Geometry: final body of the model. Coordinates: model frame, mm. Face numbers are marked on the shaded views. A direction names the side the tool comes from. Give positions to 0.01 mm unless a question says otherwise; leave off trailing zeros. Write each loop counter-clockwise with the first axis right and the second up, starting at its lowest first coordinate (ties: lowest second). Pieces come first, ordered by that corner, then holes. Notation, with made-up numbers: (60, -1.5) - (84, -1.5) arc R11 cw to (84, 14.5) - close; hole circle Ø7 at (20, 14). An arc over 180 degrees is marked (long way). Use CSV: the item, a comma, the result in double quotes. Start each with the question number.
(1) Section D-D on y = 23. Output: boundary loops of the cut face in (x, z), and give its area (3 significant figures).
(2) First-contact query: pin 1 Ø1.5 at (x, y) = (-15.5, 48.5) entering from +Z; pin 2 Ø10 at (y, z) = (23.5, 8) entering from -X; pin 3 Ø2 at (x, z) = (-3, -15.5) entering from +Y; pin 4 Ø4 at (y, z) = (7.5, -24.5) entering from -X. Flat tips, straight axial feed; report the tip coordinate or a pass-through.
(3) Draft query along Y for the marked faces 1, 2 and 3. Return one class per face: released by +Y, released by -Y, zero draft, split by the parting line, or undercut.
(4) Section A-A on z = -24. Output: boundary loops of the cut face in (x, y).
(5) Section C-C on x = 0. Output: boundary loops of the cut face in (y, z), and give its area (3 significant figures).
(6) Line query: probe 1 along Y at (x, z) = (-17.5, 5.5); probe 2 along Z at (x, y) = (4, 13.5); probe 3 along Y at (x, z) = (10, 0). Output: solid intervals per line, ascending. Write a range as [from, to].
(7) Reachability of the marked faces 4, 5, 6 and 7 from +Z, -Z, +X, -X, +Y, -Y: full face, straight path, thin tool, end or side. Return the list, or none.
(8) Section B-B on z = 0. Output: boundary loops of the cut face in (x, y), and give its area (3 significant figures).
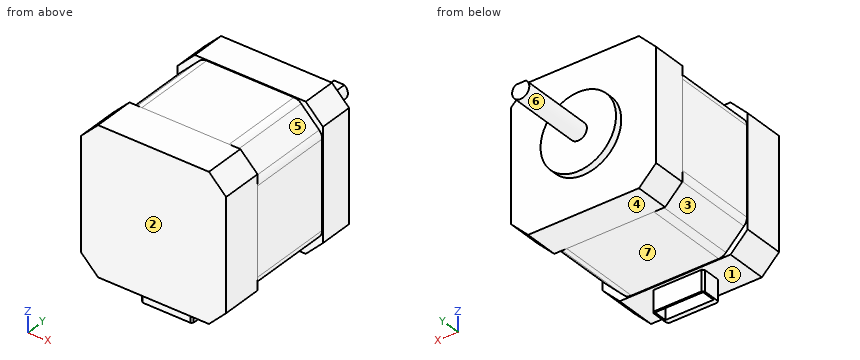
Autodesk Inventor part; units mm, degrees
ref_plane "YZ Plane" through (0, 0, 0) normal (1, 0, 0) x (0, 1, 0)
ref_plane "XZ Plane" through (0, 0, 0) normal (0, 1, 0) x (-1, 0, 0)
ref_plane "XY Plane" through (0, 0, 0) normal (0, 0, 1) x (1, 0, 0)
sketch "Эскиз1" plane through (0, 0, 0) normal (0, 1, 0) x (-1, 0, 0)
  line L0 (16.15, 21.15) -> (-16.15, 21.15)
  line L1 (-21.15, 16.15) -> (-21.15, -16.15)
  line L2 (-16.15, -21.15) -> (16.15, -21.15)
  line L3 (21.15, -16.15) -> (21.15, 16.15)
  line L4 (21.15, 21.15) -> (-21.15, -21.15) construction
  line L5 (-21.15, 21.15) -> (21.15, -21.15) construction
  line L6 (16.15, -21.15) -> (21.15, -16.15)
  line L7 (21.15, 16.15) -> (16.15, 21.15)
  line L8 (-16.15, 21.15) -> (-21.15, 16.15)
  line L9 (-21.15, -16.15) -> (-16.15, -21.15)
  point P0 (0, 0)
  dimension "d0" = 42.3
  dimension "d1" = 5
  dimension "d2" = 5
  dimension "d3" = 5
  dimension "d4" = 5
  dimension "d5" = 5
  dimension "d6" = 5
  dimension "d7" = 5
  dimension "d8" = 5
extrude "Выдавливание1" add sketch "Эскиз1" along normal blind 12
sketch "Эскиз2" plane through (0, 12, 0) normal (0, 1, 0) x (1, 0, 0)
  line L0 (13.95, -20.95) -> (-13.95, -20.95)
  line L1 (-20.95, -13.95) -> (-20.95, 13.95)
  line L2 (-13.95, 20.95) -> (13.95, 20.95)
  line L3 (20.95, 13.95) -> (20.95, -13.95)
  line L4 (20.95, -20.95) -> (-20.95, 20.95) construction
  line L5 (-20.95, -20.95) -> (20.95, 20.95) construction
  line L6 (-16.15, -21.15) -> (16.15, -21.15)
  line L7 (-13.95, -20.95) -> (-20.95, -13.95)
  line L8 (-20.95, 13.95) -> (-13.95, 20.95)
  line L9 (13.95, 20.95) -> (20.95, 13.95)
  line L10 (20.95, -13.95) -> (13.95, -20.95)
  point P0 (0, 0)
  dimension "d23" = 0.2
  dimension "d24" = 7
  dimension "d25" = 7
  dimension "d26" = 7
  dimension "d27" = 7
  dimension "d28" = 7
  dimension "d29" = 7
  dimension "d30" = 7
  dimension "d31" = 7
extrude "Выдавливание2" add sketch "Эскиз2" along normal blind 25
sketch "Эскиз3" plane through (0, 37, 0) normal (0, 1, 0) x (1, 0, 0)
  line L0 (-16.15, 21.15) -> (-21.15, 16.15)
  line L1 (16.15, 21.15) -> (-16.15, 21.15)
  line L2 (21.15, 16.15) -> (16.15, 21.15)
  line L3 (21.15, -16.15) -> (21.15, 16.15)
  line L4 (16.15, -21.15) -> (21.15, -16.15)
  line L5 (-16.15, -21.15) -> (16.15, -21.15)
  line L6 (-21.15, -16.15) -> (-16.15, -21.15)
  line L7 (-21.15, 16.15) -> (-21.15, -16.15)
  point P0 (0, 0)
extrude "Выдавливание3" add sketch "Эскиз3" along normal blind 10
fillet "Сопряжение1" radius 3 8 edges at (13.95, 24.5, 20.95) (20.95, 24.5, 13.95) (20.95, 24.5, -13.95) (13.95, 24.5, -20.95) (-13.95, 24.5, -20.95) (-20.95, 24.5, -13.95) (-20.95, 24.5, 13.95) (-13.95, 24.5, 20.95)
sketch "Эскиз4" plane through (0, 47, 0) normal (0, 1, 0) x (1, 0, 0)
  circle A0 centre (0, 0) radius 11
  dimension "d33" = 22
extrude "Выдавливание4" add sketch "Эскиз4" along normal blind 2
sketch "Эскиз5" plane through (0, 49, 0) normal (0, 1, 0) x (1, 0, 0)
  arc A0 (1.5, -2) -> (-1.5, -2) centre (0, 0) ccw
  line L0 (1.5, -2) -> (-1.5, -2)
  dimension "d36" = 2.5
  dimension "d37" = 2
extrude "Выдавливание5" add sketch "Эскиз5" along normal blind 22
sketch "Эскиз6" plane through (16.15, 0, -21.15) normal (0, 0, -1) x (-1, 0, 0)
  line L0 (0, 0) -> (32.3, 0)
  line L1 (8.65, 11) -> (23.65, 11)
  line L2 (23.65, 11) -> (23.65, 5)
  line L3 (23.65, 5) -> (8.65, 5)
  line L4 (8.65, 5) -> (8.65, 11)
  point P0 (16.15, 0)
  point P1 (16.15, 0)
  point P2 (16.15, 5)
  point P3 (16.15, 0)
  dimension "d67" = 15
  dimension "d68" = 6
  dimension "d69" = 5
extrude "Выдавливание6" add sketch "Эскиз6" along normal blind 6
sketch "Эскиз9" plane through (16.15, 0, -27.15) normal (0, 0, -1) x (-1, 0, 0)
  line L0 (9.15, 10.5) -> (23.15, 10.5)
  line L1 (23.15, 10.5) -> (23.15, 6.5)
  line L2 (23.15, 6.5) -> (9.15, 6.5)
  line L3 (9.15, 6.5) -> (9.15, 10.5)
  line L4 (23.65, 5) -> (23.65, 11)
  line L5 (23.65, 11) -> (8.65, 11)
  point P0 (16.15, 0)
  point P1 (16.15, 6.5)
  dimension "d70" = 0.5
  dimension "d71" = 0.5
  dimension "d72" = 4
extrude "Выдавливание8" cut sketch "Эскиз9" against normal blind 4
chamfer "Фаска1" distance 0.5 angle 45 4 edges at (7.5, 11, -24.15) (7.5, 5, -24.15) (-7.5, 11, -24.15) (-7.5, 5, -24.15)
equation "\"d2\" = d1"
equation "\"d3\" = d1"
equation "\"d4\" = d3"
equation "\"d5\" = d1"
equation "\"d6\" = d5"
equation "\"d7\" = d1"
equation "\"d8\" = d7"
equation "\"d25\" = d24"
equation "\"d26\" = d24"
equation "\"d27\" = d26"
equation "\"d28\" = d24"
equation "\"d29\" = d28"
equation "\"d30\" = d24"
equation "\"d31\" = d30"
properties part number "42BYGH47" material "Сталь, мягкая"
Check values:
1,outline,"(-20.95, -12.71) arc R3 ccw to (-20.07, -14.83) - (-14.83, -20.07) arc R3 ccw to (-12.71, -20.95) - (12.71, -20.95) arc R3 ccw to (14.83, -20.07) - (20.07, -14.83) arc R3 ccw to (20.95, -12.71) - (20.95, 12.71) arc R3 ccw to (20.07, 14.83) - (14.83, 20.07) arc R3 ccw to (12.71, 20.95) - (-12.71, 20.95) arc R3 ccw to (-14.83, 20.07) - (-20.07, 14.83) arc R3 ccw to (-20.95, 12.71) - close"
1,area,"1,660 mm²"
2,pin 1,"passes through"
2,pin 2,"stops at x = -20.95"
2,pin 3,"stops at y = 47"
2,pin 4,"stops at x = -7.5"
3,face 1,"zero draft"
3,face 2,"released by -Y"
3,face 3,"undercut"
4,outline,"(-7.5, 5.5) - (-7, 5) - (7, 5) - (7.5, 5.5) - (7.5, 10.5) - (7, 11) - (-7, 11) - (-7.5, 10.5) - close; hole (-7, 6.5) - (7, 6.5) - (7, 10.5) - (-7, 10.5) - close"
5,outline,"(0, -21.15) - (5, -21.15) - (5, -27.15) - (6.5, -27.15) - (6.5, -23.15) - (10.5, -23.15) - (10.5, -27.15) - (11, -27.15) - (11, -21.15) - (12, -21.15) - (12, -20.95) - (37, -20.95) - (37, -21.15) - (47, -21.15) - (47, -11) - (49, -11) - (49, -2.5) - (71, -2.5) - (71, 2) - (49, 2) - (49, 11) - (47, 11) - (47, 21.15) - (37, 21.15) - (37, 20.95) - (12, 20.95) - (12, 21.15) - (0, 21.15) - close"
5,area,"2,140 mm²"
6,probe 1,"y = [0, 47]"
6,probe 2,"z = [-20.95, 20.95]"
6,probe 3,"y = [0, 49]"
7,face 4,"-Z, +X, -X, +Y"
7,face 5,"+Z, +X"
7,face 6,"+Y"
7,face 7,"-Z, +X, -X"
8,outline,"(-21.15, 0) - (21.15, 0) - (21.15, 12) - (20.95, 12) - (20.95, 37) - (21.15, 37) - (21.15, 47) - (11, 47) - (11, 49) - (2.5, 49) - (2.5, 71) - (-2.5, 71) - (-2.5, 49) - (-11, 49) - (-11, 47) - (-21.15, 47) - (-21.15, 37) - (-20.95, 37) - (-20.95, 12) - (-21.15, 12) - close"
8,area,"2,130 mm²"
